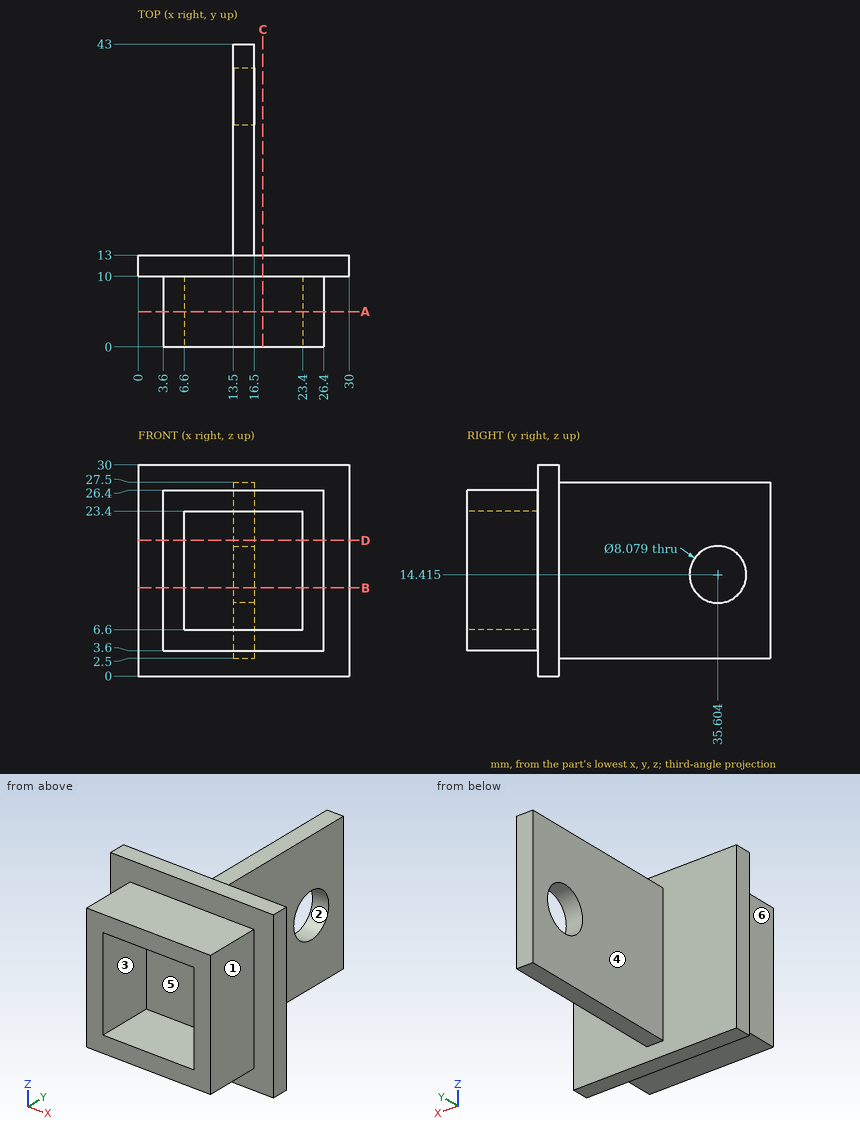
Job drawing, mm, ordinate dimensions from the low corner. One solid piece. A direction names the side the tool comes from. Coordinates: 2 decimals unless noted, no trailing zeros. Write each loop counter-clockwise with the first axis right and the second up, starting at its lowest first coordinate (ties: lowest second). Pieces come first, ordered by that corner, then holes. Notation, with made-up numbers: M 50,-5.5 L 97,-5.5 A18 cw 97,24.5 Z; hole C -21,79.5 d7. An arc over 180 degrees is marked long. Answer as a JSON object with one key per item and string values. Group by question number.
1) Mould opens along X. For the marked faces 1, 2 and 3 say: +X half, -X half, draft (parallel to the pull), parting line (faces both ways), or undercut.
2) Wall check: line 1 (X direction, y = 9, z = 7.5); line 2 (Y direction, x = 10, z = 12.25). Give the ranges that are in metal, low to high. Write a range as from..to.
3) Saw through at C-C (x = 17.75). Write the cut outline in (y, z), plus the area to 3 significant figures.
4) Tool access for the marked faces 4, 5 and 6: list every direction of +Z, -Z, +X, -X, +Y, -Y with a clear straight run to the whole face (end or side of a thin tool).
5) Pin check, flat tips, straight feed: pin 1 Ø3.5 at (x, y) = (15.5, 30.5) entering from -Z; pin 2 Ø9.5 at (y, z) = (35.6, 14.42) entering from -X; pin 3 Ø1 at (x, y) = (5.5, 5) entering from +Z. Stop position of each tip, or through.
6) Saw through at D-D (z = 19.25). Write the cut outline in (x, y), plus the area to 3 significant figures.
7) Saw through at B-B (z = 12.5). Write the cut outline in (x, y).
8) Saw through at A-A (y = 5). Write the cut outline in (x, z).
Values follow:
{
 "1": {"face 1": "+X half", "face 2": "draft", "face 3": "undercut"},
 "2": {"line 1": "x = 3.6..6.6, 23.4..26.4", "line 2": "y = 10..13"},
 "3": {"outline": "M 0,3.6 L 10,3.6 L 10,0 L 13,0 L 13,30 L 10,30 L 10,26.4 L 0,26.4 L 0,23.4 L 10,23.4 L 10,6.6 L 0,6.6 Z", "area": "150 mm2"},
 "4": {"face 4": "+Z, -Z, -X, +Y", "face 5": "-Y", "face 6": "+Z, -Z, -X, -Y"},
 "5": {"pin 1": "stops at z = 2.5", "pin 2": "stops at x = 13.5", "pin 3": "stops at z = 26.4"},
 "6": {"outline": "M 0,10 L 3.6,10 L 3.6,0 L 6.6,0 L 6.6,10 L 23.4,10 L 23.4,0 L 26.4,0 L 26.4,10 L 30,10 L 30,13 L 16.5,13 L 16.5,43 L 13.5,43 L 13.5,13 L 0,13 Z", "area": "240 mm2"},
 "7": {"outline": "M 0,10 L 3.6,10 L 3.6,0 L 6.6,0 L 6.6,10 L 23.4,10 L 23.4,0 L 26.4,0 L 26.4,10 L 30,10 L 30,13 L 16.5,13 L 16.5,32.05 L 13.5,32.05 L 13.5,13 L 0,13 Z; M 13.5,39.16 L 16.5,39.16 L 16.5,43 L 13.5,43 Z"},
 "8": {"outline": "M 3.6,3.6 L 26.4,3.6 L 26.4,26.4 L 3.6,26.4 Z; hole M 6.6,6.6 L 23.4,6.6 L 23.4,23.4 L 6.6,23.4 Z"}
}
